Autodesk Inventor part; units mm, degrees
ref_plane "YZ Plane" through (0, 0, 0) normal (1, 0, 0) x (0, 1, 0)
ref_plane "XZ Plane" through (0, 0, 0) normal (0, 1, 0) x (-1, 0, 0)
ref_plane "XY Plane" through (0, 0, 0) normal (0, 0, 1) x (1, 0, 0)
sketch "Sketch1" plane through (0, 0, 0) normal (0, 1, 0) x (-1, 0, 0)
  line L0 (0, 0) -> (0, -36)
  line L1 (0, -36) -> (-40, -36)
  line L2 (-40, -36) -> (-40, 0)
  line L3 (-40, 0) -> (0, 0)
  line L4 (0, -18) -> (-40, -18) construction
  line L5 (-20, 0) -> (-20, -36) construction
  circle A0 centre (-36, -12) radius 1.75
  circle A1 centre (-36, -24) radius 1.75
  circle A2 centre (-4, -10.7051) radius 1.75
  circle A3 centre (-4, -25.75) radius 1.75
  circle A4 centre (-28, -5) radius 1.75
  circle A5 centre (-12, -5.4968) radius 1.75
  circle A6 centre (-28, -31) radius 1.75
  circle A7 centre (-12, -29.25) radius 1.75
  line L6 (-20, -18) -> (-18.5, -18) construction
  line L7 (-20, -18) -> (-21.5, -18) construction
  line L8 (-18.5, -12) -> (-18.5, -25.5) construction
  line L9 (-18.5, -12) -> (-18.5, -25.5)
  line L10 (-18.5, -25.5) -> (-21.5, -25.5)
  line L11 (-21.5, -25.5) -> (-21.5, -12)
  line L12 (-21.5, -12) -> (-18.5, -12)
  line L13 (-18.5, -16.9522) -> (-17, -16.9522) construction
  line L14 (-21.5, -16.9522) -> (-23, -16.9522) construction
  line L15 (-23, -12) -> (-23, -25.5) construction
  line L16 (-23, -12) -> (-23, -25.5)
  line L17 (-23, -25.5) -> (-25.5, -25.5)
  line L18 (-25.5, -25.5) -> (-25.5, -12)
  line L19 (-25.5, -12) -> (-23, -12)
  line L20 (-17, -12) -> (-17, -25.5)
  line L21 (-17, -25.5) -> (-14.5, -25.5)
  line L22 (-14.5, -25.5) -> (-14.5, -12)
  line L23 (-14.5, -12) -> (-17, -12)
  dimension "d0" = 36
  dimension "d1" = 40
  dimension "d4" = 3.5
  dimension "d5" = 6
  dimension "d7" = 3.5
  dimension "d8" = 3.5
  dimension "d14" = 32
  dimension "d15" = 4
  dimension "d16" = 4
  dimension "d17" = 4
  dimension "d19" = 3.5
  dimension "d20" = 3.5
  dimension "d21" = 3.5
  dimension "d23" = 5
  dimension "d24" = 5
  dimension "d28" = 16
  dimension "d29" = 12
  dimension "d30" = 3.5
  dimension "d31" = 16
  dimension "d32" = 10.7051
  dimension "d33" = 25.75
  dimension "d34" = 5.4968
  dimension "d35" = 29.25
  dimension "d42" = 3
  dimension "d45" = 1.5
  dimension "d53" = 2.5
  dimension "d54" = 90
  dimension "d56" = 23
  dimension "d61" = 12
  dimension "d62" = 12
  dimension "d66" = 13.5
  dimension "d67" = 2.5
  dimension "d70" = 14.5
  dimension "d71" = 4.9522
  dimension "d72" = 24
  dimension "d73" = 13.5
  dimension "d74" = 4.9522
  dimension "d75" = 0
  dimension "d76" = 13.5
  dimension "d77" = 17
  dimension "d78" = 18.5
  dimension "d79" = 21.5
  dimension "d80" = 23
  dimension "d81" = 12
extrude "Extrusion3" add sketch "Sketch1" along normal blind 1
properties part number "valvle plate"
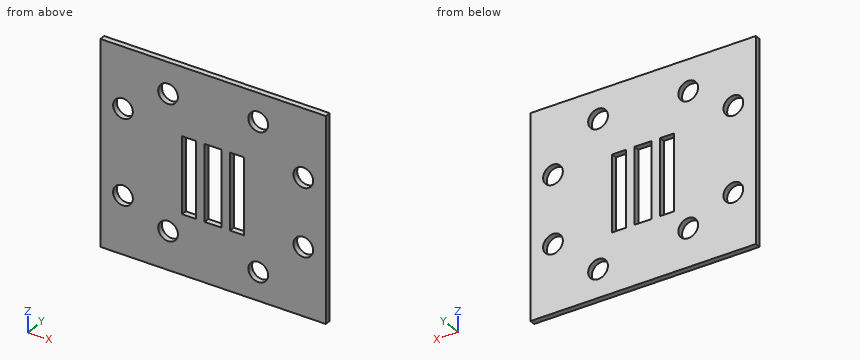
Verification items for the finished model (mm, model axes). Round coordinates to 2 decimals unless told otherwise and drop trailing zeros. Write each loop counter-clockwise with the first axis right and the second up, starting at its lowest first coordinate (ties: lowest second). Pieces come first, ordered by that corner, then holes. Notation, with made-up numbers: (11.5, -39.75) -> (26.5, -39.75) arc R5 ccw to (26.5, -31.75) -> close; hole circle Ø11 at (-30, -12). An arc over 180 degrees is marked (long way). Write each question's results on one line, items separated by ' | '. Start each with the question number.
1. Material ranges on probe 1 along Z at (x, y) = (36, 0.6); probe 2 along Z at (x, y) = (4, 0.2); probe 3 along X at (y, z) = (0.15, -21), recorded low to high. Write a range as from..to.
2. Cross-section at C-C (y = 0.6). Count the separate pieces of the cut face and the enclosed holes in it, then the cut area to 3 significant figures.
3. Cross-section at B-B (z = -15). Enter the section's corners in (x, y).
4. Cross-section at A-A (x = 28). Enter the section's corners in (y, z).
5. Cross-section at D-D (z = -5). Enter the section's corners in (x, y), then the cut area to 3 significant figures.
Solutions:
1) probe 1: z = -36..-25.75, -22.25..-13.75, -10.25..0 | probe 2: z = -36..-27.5, -24..-12.46, -8.96..0 | probe 3: x = 0..14.5, 17..18.5, 21.5..23, 25.5..40
2) separate pieces: 1 | enclosed holes: 11 | area: 1,260 mm2
3) outline: (0, 0) -> (14.5, 0) -> (14.5, 1) -> (0, 1) -> close; (17, 0) -> (18.5, 0) -> (18.5, 1) -> (17, 1) -> close; (21.5, 0) -> (23, 0) -> (23, 1) -> (21.5, 1) -> close; (25.5, 0) -> (40, 0) -> (40, 1) -> (25.5, 1) -> close
4) outline: (0, -36) -> (1, -36) -> (1, -32.75) -> (0, -32.75) -> close; (0, -29.25) -> (1, -29.25) -> (1, -6.75) -> (0, -6.75) -> close; (0, -3.25) -> (1, -3.25) -> (1, 0) -> (0, 0) -> close
5) outline: (0, 0) -> (10.32, 0) -> (10.32, 1) -> (0, 1) -> close; (13.68, 0) -> (26.25, 0) -> (26.25, 1) -> (13.68, 1) -> close; (29.75, 0) -> (40, 0) -> (40, 1) -> (29.75, 1) -> close | area: 33.1 mm2
